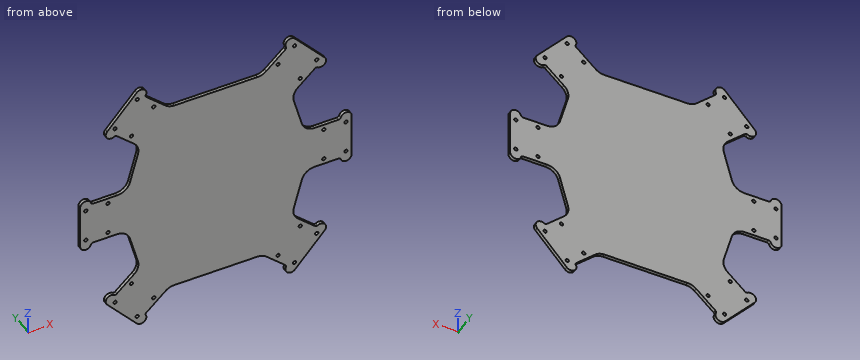
```python
from build123d import *

# Parameters (mm, degrees)
SKETCH2_R               = 1.5
BOSS_EXTRUDE1_DEPTH     = 3
SKETCH7_R               = 1.5
CUT_EXTRUDE4_DEPTH      = 10
MIRROR2_COPY_1_SKETCH_R = 1.5
MIRROR2_COPY_1_DEPTH    = 10
CUT_EXTRUDE5_START      = -10
SKETCH8_R               = 1.5
CUT_EXTRUDE5_DEPTH      = 10


with BuildPart() as part:
    # Sketch2 → Boss-Extrude1 (new body)
    with BuildSketch(Plane(origin=(0, 0, 0), x_dir=(1, 0, 0), z_dir=(0, 1, 0))):
        with BuildLine():
            Line((77.604131862, 28.818122204), (70.352023373, 55.1894258))
            ThreePointArc((70.352023373, 55.1894258), (70.409142384, 61.75403485), (73.912058214, 67.306235788))
            Line((73.912058214, 67.306235788), (89.448492578, 81.235106792))
            ThreePointArc((89.448492578, 81.235106792), (90.603066053, 81.737789877), (91.829194878, 81.450843369))
            ThreePointArc((91.829194878, 81.450843369), (98.283456403, 82.511045735), (98.166159929, 89.050752337))
            Line((98.166159929, 89.050752337), (71.464727022, 118.833859641))
            ThreePointArc((71.464727022, 118.833859641), (64.976597411, 119.661926694), (63.220516764, 113.361315481))
            ThreePointArc((63.220516764, 113.361315481), (63.372367291, 112.111246838), (62.747059671, 111.018214097))
            Line((62.747059671, 111.018214097), (45.510429872, 95.565067809))
            ThreePointArc((45.510429872, 95.565067809), (41.788403765, 93.292431435), (37.5, 92.5))
            Line((37.5, 92.5), (-37.5, 92.5))
            ThreePointArc((-37.5, 92.5), (-41.788403765, 93.292431435), (-45.510429872, 95.565067809))
            Line((-45.510429872, 95.565067809), (-62.747059671, 111.018214097))
            ThreePointArc((-62.747059671, 111.018214097), (-63.372367291, 112.111246838), (-63.220516764, 113.361315481))
            ThreePointArc((-63.220516764, 113.361315481), (-64.976597411, 119.661926694), (-71.464727022, 118.833859641))
            Line((-71.464727022, 118.833859641), (-98.166159929, 89.050752337))
            ThreePointArc((-98.166159929, 89.050752337), (-98.283456403, 82.511045735), (-91.829194878, 81.450843369))
            ThreePointArc((-91.829194878, 81.450843369), (-90.603066053, 81.737789877), (-89.448492578, 81.235106792))
            Line((-89.448492578, 81.235106792), (-73.912058214, 67.306235788))
            ThreePointArc((-73.912058214, 67.306235788), (-70.409142384, 61.75403485), (-70.352023373, 55.1894258))
            Line((-70.352023373, 55.1894258), (-77.604131862, 28.818122204))
            ThreePointArc((-77.604131862, 28.818122204), (-81.900757615, 22.455825506), (-89.174596575, 20))
            Line((-89.174596575, 20), (-110.791796068, 20))
            ThreePointArc((-110.791796068, 20), (-111.987024677, 20.396432549), (-112.708425763, 21.428571429))
            ThreePointArc((-112.708425763, 21.428571429), (-118.221847911, 24.947619184), (-122.5, 20))
            Line((-122.5, 20), (-122.5, -20))
            ThreePointArc((-122.5, -20), (-118.221847911, -24.947619184), (-112.708425762, -21.428571429))
            ThreePointArc((-112.708425762, -21.428571429), (-111.987024677, -20.396432549), (-110.791796067, -20))
            Line((-110.791796067, -20), (-89.174596575, -20))
            ThreePointArc((-89.174596575, -20), (-81.900757615, -22.455825506), (-77.604131862, -28.818122204))
            Line((-77.604131862, -28.818122204), (-70.352023373, -55.1894258))
            ThreePointArc((-70.352023373, -55.1894258), (-70.409142384, -61.75403485), (-73.912058214, -67.306235788))
            Line((-73.912058214, -67.306235788), (-89.448492578, -81.235106792))
            ThreePointArc((-89.448492578, -81.235106792), (-90.603066053, -81.737789877), (-91.829194878, -81.450843369))
            ThreePointArc((-91.829194878, -81.450843369), (-98.283456403, -82.511045735), (-98.166159929, -89.050752337))
            Line((-98.166159929, -89.050752337), (-71.464727022, -118.833859641))
            ThreePointArc((-71.464727022, -118.833859641), (-64.976597411, -119.661926694), (-63.220516764, -113.361315481))
            ThreePointArc((-63.220516764, -113.361315481), (-63.372367291, -112.111246838), (-62.747059671, -111.018214097))
            Line((-62.747059671, -111.018214097), (-45.510429872, -95.565067809))
            ThreePointArc((-45.510429872, -95.565067809), (-41.788403765, -93.292431435), (-37.5, -92.5))
            Line((-37.5, -92.5), (37.5, -92.5))
            ThreePointArc((37.5, -92.5), (41.788403765, -93.292431435), (45.510429872, -95.565067809))
            Line((45.510429872, -95.565067809), (62.747059671, -111.018214097))
            ThreePointArc((62.747059671, -111.018214097), (63.372367291, -112.111246838), (63.220516764, -113.361315481))
            ThreePointArc((63.220516764, -113.361315481), (64.976597411, -119.661926694), (71.464727022, -118.833859641))
            Line((71.464727022, -118.833859641), (98.166159929, -89.050752337))
            ThreePointArc((98.166159929, -89.050752337), (98.283456403, -82.511045735), (91.829194878, -81.450843369))
            ThreePointArc((91.829194878, -81.450843369), (90.603066053, -81.737789877), (89.448492578, -81.235106792))
            Line((89.448492578, -81.235106792), (73.912058214, -67.306235788))
            ThreePointArc((73.912058214, -67.306235788), (70.409142384, -61.75403485), (70.352023373, -55.1894258))
            Line((70.352023373, -55.1894258), (77.604131862, -28.818122204))
            ThreePointArc((77.604131862, -28.818122204), (81.900757615, -22.455825506), (89.174596575, -20))
            Line((89.174596575, -20), (110.791796067, -20))
            ThreePointArc((110.791796067, -20), (111.987024677, -20.396432549), (112.708425762, -21.428571429))
            ThreePointArc((112.708425762, -21.428571429), (118.221847911, -24.947619184), (122.5, -20))
            Line((122.5, -20), (122.5, 20))
            ThreePointArc((122.5, 20), (118.221847911, 24.947619184), (112.708425763, 21.428571429))
            ThreePointArc((112.708425763, 21.428571429), (111.987024677, 20.396432549), (110.791796068, 20))
            Line((110.791796068, 20), (89.174596575, 20))
            ThreePointArc((89.174596575, 20), (81.900757615, 22.455825506), (77.604131862, 28.818122204))
        make_face()
        with Locations(Location((-91.038580411, 89.375883412, 0), (0, 0, 270))):
            Circle(SKETCH2_R, mode=Mode.SUBTRACT)
        with Locations(Location((-71.012505731, 111.713213891, 0), (0, 0, 90))):
            Circle(SKETCH2_R, mode=Mode.SUBTRACT)
        with Locations(Location((91.038580411, 89.375883412, 0), (0, 0, 90))):
            Circle(SKETCH2_R, mode=Mode.SUBTRACT)
        with Locations(Location((71.012505731, 111.713213891, 0), (0, 0, 270))):
            Circle(SKETCH2_R, mode=Mode.SUBTRACT)
        with Locations(Location((91.038580411, -89.375883412, 0), (0, 0, 270))):
            Circle(SKETCH2_R, mode=Mode.SUBTRACT)
        with Locations(Location((71.012505731, -111.713213891, 0), (0, 0, 90))):
            Circle(SKETCH2_R, mode=Mode.SUBTRACT)
        with Locations(Location((-71.012505731, -111.713213891, 0), (0, 0, 270))):
            Circle(SKETCH2_R, mode=Mode.SUBTRACT)
        with Locations(Location((-91.038580411, -89.375883412, 0), (0, 0, 90))):
            Circle(SKETCH2_R, mode=Mode.SUBTRACT)
        with Locations(Location((-117.41, -15, 0), (0, 0, 270))):
            Circle(SKETCH2_R, mode=Mode.SUBTRACT)
        with Locations(Location((-117.41, 15, 0), (0, 0, 90))):
            Circle(SKETCH2_R, mode=Mode.SUBTRACT)
        with Locations(Location((117.41, -15, 0), (0, 0, 90))):
            Circle(SKETCH2_R, mode=Mode.SUBTRACT)
        with Locations(Location((117.41, 15, 0), (0, 0, 270))):
            Circle(SKETCH2_R, mode=Mode.SUBTRACT)
    extrude(amount=BOSS_EXTRUDE1_DEPTH)

    # Sketch7 → Cut-Extrude4 (cut)
    with BuildSketch(Plane(origin=(0, 3, 0), x_dir=(1, 0, 0), z_dir=(0, 1, 0))):
        with Locations(Location((-76.147026759, 76.025166959, 0), (0, 0, 270))):
            Circle(SKETCH7_R)
        with Locations(Location((-56.120952079, 98.362497437, 0), (0, 0, 270))):
            Circle(SKETCH7_R)
    cut_extrude4 = extrude(amount=-CUT_EXTRUDE4_DEPTH, mode=Mode.SUBTRACT)

    # Mirror1: Cut-Extrude4 across plane
    add(cut_extrude4.mirror(Plane(origin=(0, 0, 0), x_dir=(0, 0, 1), z_dir=(1, 0, 0))), mode=Mode.SUBTRACT)

    # Mirror2: Cut-Extrude4 across plane
    add(cut_extrude4.mirror(Plane.XY), mode=Mode.SUBTRACT)

    # Mirror2 copy 1 sketch → Mirror2 copy 1 (cut)
    with BuildSketch(Plane(origin=(0, 3, 0), x_dir=(-1, 0, 0), z_dir=(0, 1, 0))):
        with Locations(Location((-76.147026759, 76.025166959, 0), (0, 0, 270))):
            Circle(MIRROR2_COPY_1_SKETCH_R)
        with Locations(Location((-56.120952079, 98.362497437, 0), (0, 0, 270))):
            Circle(MIRROR2_COPY_1_SKETCH_R)
    extrude(amount=-MIRROR2_COPY_1_DEPTH, mode=Mode.SUBTRACT)

    # Sketch8 → Cut-Extrude5 (cut)
    with BuildSketch(Plane(origin=(0, 3, 0), x_dir=(1, 0, 0), z_dir=(0, 1, 0)).offset(CUT_EXTRUDE5_START)):
        with Locations(Location((-117.41, 15, 0), (0, 0, 90))):
            Circle(SKETCH8_R)
        with Locations(Location((-117.41, -15, 0), (0, 0, 270))):
            Circle(SKETCH8_R)
        with Locations(Location((-97.41, -15, 0), (0, 0, 270))):
            Circle(SKETCH8_R)
        with Locations(Location((-97.41, 15, 0), (0, 0, 270))):
            Circle(SKETCH8_R)
    cut_extrude5 = extrude(amount=CUT_EXTRUDE5_DEPTH, mode=Mode.SUBTRACT)

    # Mirror3: Cut-Extrude5 across plane
    add(cut_extrude5.mirror(Plane(origin=(0, 0, 0), x_dir=(0, 0, 1), z_dir=(1, 0, 0))), mode=Mode.SUBTRACT)


solid = part.part
```
Could you check a few things on this model? Use its own coordinates, in mm. Round coordinates to 2 decimals unless told otherwise and drop trailing zeros. Write each loop counter-clockwise with the first axis right and the second up, starting at its lowest first coordinate (ties: lowest second). Pieces come first, ordered by that corner, then holes.
(1) Suppose I cut it at A-A on y = 1.25. State how many separate pieces and enclosed holes the cut face has, and give its area (3 significant figures).
Findings below:
separate pieces: 1
enclosed holes: 24
area: 35,800 mm2
(2) Suppose I cut it at B-B on x = -28. Write out the boundary of the cut face in (y, z), and give its area (3 significant figures).
Findings below:
outline: (0, -92.5) - (3, -92.5) - (3, 92.5) - (0, 92.5) - close
area: 555 mm2
(3) If I drill on probe 1 along Z at (x, y) = (-92, 1.5); probe 2 along Z at (x, y) = (-93.5, 0.9); probe 3 along Z at (x, y) = (13.5, 1.3), over which ranges is the centre line in solid material (lowest first)?
Findings below:
probe 1: z = -95.93 to -90.53, -88.22 to -81.35, -20 to 20, 81.35 to 88.22, 90.53 to 95.93
probe 2: z = -94.26 to -80.8, -20 to 20, 80.8 to 94.26
probe 3: z = -92.5 to 92.5
(4) Suppose I cut it at C-C on z = -42.5. Write out the boundary of the cut face in (x, y).
Findings below:
outline: (-73.84, 0) - (73.84, 0) - (73.84, 3) - (-73.84, 3) - close
(5) For pin 1 (1.5 mm diameter, centred on x = 2.5, y = 1.5, fed in from +Z); pin 2 (0.9 mm diameter, centred on x = -104.5, y = 1.5, fed in from -Z); pin 3 (1 mm diameter, centred on y = 2.5, z = -72, fed in from -X), each with a flat end and sliding along its axis, tell me the tip position at first contact or that it passes through.
Findings below:
pin 1: stops at z = 92.5
pin 2: stops at z = -20
pin 3: stops at x = -79.71
